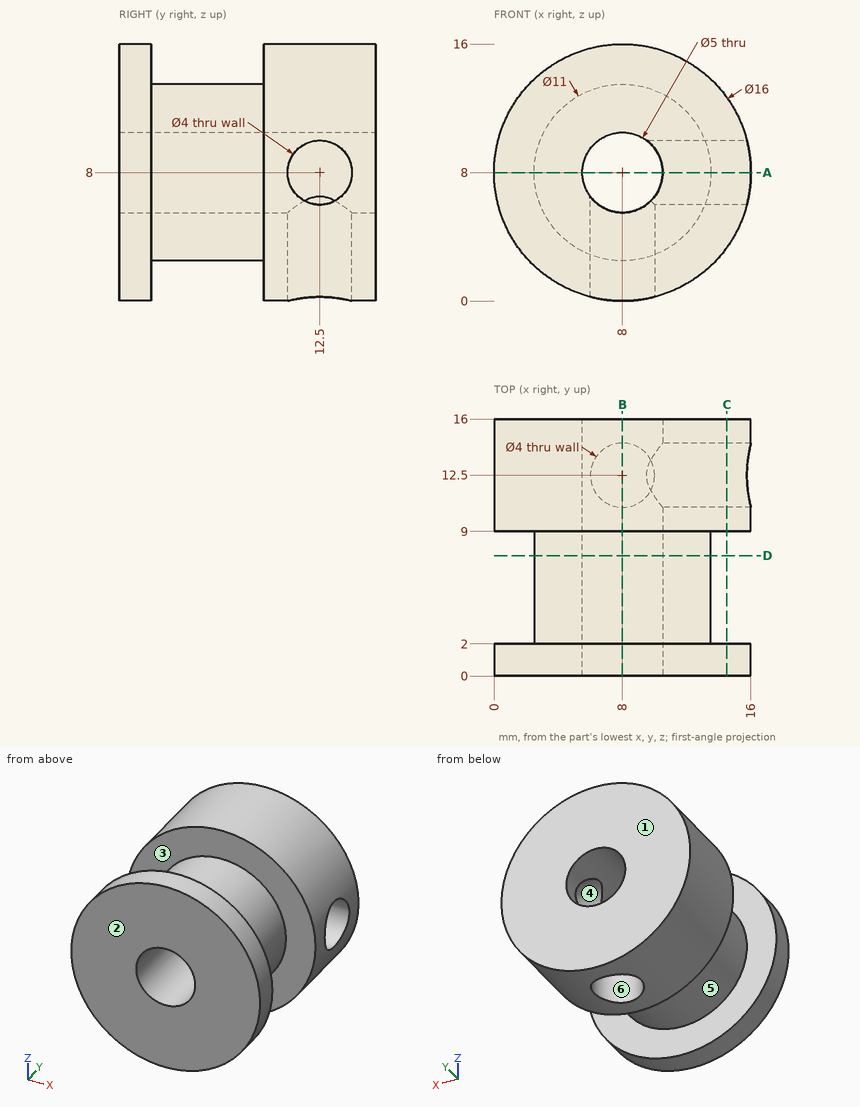
Part print with two shaded views. Sizes in mm from the minimum x, y, z corner. A direction names the side the tool comes from. Give positions to 0.01 mm unless a question says otherwise; leave off trailing zeros. Write each loop counter-clockwise with the first axis right and the second up, starting at its lowest first coordinate (ties: lowest second). Pieces come first, ordered by that corner, then holes.
1) Cut at D-D on y = 7.5. Write the cut outline in (x, z), then the cut area to 3 significant figures.
Resolved:
outline: circle Ø11 at (8, 8); hole circle Ø5 at (8, 8)
area: 75.4 mm2
2) Which spindle directions (+Z, -Z, +X, -X, +Y, -Y) get a long thin tool onto all of the face, cutting with end or side? Do the marked faces 4, 5 and 6. Say none if no direction does.
Resolved:
face 4: +X
face 5: none
face 6: -Z
3) Cut at A-A on z = 8. Write the cut outline in (x, y).
Resolved:
outline: (0, 0) - (5.5, 0) - (5.5, 16) - (0, 16) - (0, 9) - (2.5, 9) - (2.5, 2) - (0, 2) - close; (10.5, 0) - (16, 0) - (16, 2) - (13.5, 2) - (13.5, 9) - (16, 9) - (16, 10.5) - (10.5, 10.5) - close; (10.5, 14.5) - (16, 14.5) - (16, 16) - (10.5, 16) - close
4) Cut at C-C on x = 14.5. Write the cut outline in (y, z).
Resolved:
outline: (0, 3.34) - (2, 3.34) - (2, 12.66) - (0, 12.66) - close; (9, 3.34) - (16, 3.34) - (16, 12.66) - (9, 12.66) - close; hole circle Ø4 at (12.5, 8)
5) Two-plate mould, pull along Y, no slides. Class the marked faces 1, 2 and 3: released by +Y, released by -Y, zero draft, split by the parting line, or undercut.
Resolved:
face 1: released by +Y
face 2: released by -Y
face 3: undercut
6) Probe L1, parallel to Y at x = 2.5, z = 13; L2, parallel to Z at x = 8, y = 10; L3, parallel to Y at x = 8, z = 4.5. List the from-to ranges inside material, lowest first.
Resolved:
L1: y = 0 to 2, 9 to 16
L2: z = 0 to 5.5, 10.5 to 16
L3: y = 0 to 10.5, 14.5 to 16
7) Pin check, flat tips, straight feed: pin 1 (2 mm diameter, centred on x = 7.5, y = 6, fed in from +Z); pin 2 (6 mm diameter, centred on y = 14, z = 3.5, fed in from +X); pin 3 (1 mm diameter, centred on y = 7, z = 12.5, fed in from +X). Stop position of each tip, or through.
Resolved:
pin 1: stops at z = 13.5
pin 2: stops at x = 15.86
pin 3: stops at x = 11.77
8) Cut at B-B on x = 8. Write the cut outline in (y, z), then the cut area to 3 significant figures.
Resolved:
outline: (0, 0) - (2, 0) - (2, 2.5) - (9, 2.5) - (9, 0) - (10.5, 0) - (10.5, 5.5) - (0, 5.5) - close; (0, 10.5) - (16, 10.5) - (16, 16) - (9, 16) - (9, 13.5) - (2, 13.5) - (2, 16) - (0, 16) - close; (14.5, 0) - (16, 0) - (16, 5.5) - (14.5, 5.5) - close
area: 119 mm2
